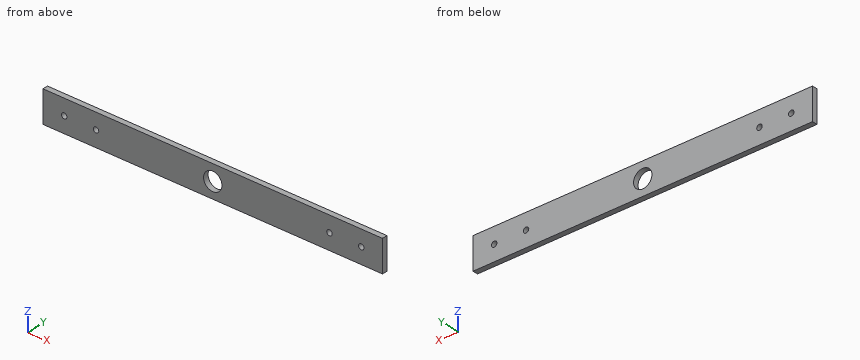
```python
from build123d import *

# Parameters (mm, degrees)
SKETCH1_W                = 406.4
SKETCH1_H                = 38.1
BOSS_EXTRUDE1_DEPTH      = 6.35
SKETCH2_R                = 11
CUT_EXTRUDE1_DEPTH       = 7.62
F_0_257_DIAMETER_HOLE1_D = 6.5278


with BuildPart() as part:
    # Sketch1 → Boss-Extrude1 (new body)
    with BuildSketch(Plane(origin=(0, 0, 0), x_dir=(1, 0, 0), z_dir=(0, 1, 0))):
        Rectangle(SKETCH1_W, SKETCH1_H)
    extrude(amount=BOSS_EXTRUDE1_DEPTH)

    # Sketch2 → Cut-Extrude1 (cut)
    with BuildSketch(Plane(origin=(0, 6.35, 0), x_dir=(1, 0, 0), z_dir=(0, 1, 0))):
        Circle(SKETCH2_R)
    extrude(amount=-CUT_EXTRUDE1_DEPTH, mode=Mode.SUBTRACT)

    # F (0.257) Diameter Hole1 (through all)
    with Locations(Plane(origin=(0, 6.35, 0), x_dir=(1, 0, 0), z_dir=(0, 1, 0))):
        with Locations((177.8, 0), (139.7, 0)):
            f_0_257_diameter_hole1 = Hole(F_0_257_DIAMETER_HOLE1_D / 2)

    # Mirror1: F (0.257) Diameter Hole1 across plane
    add(f_0_257_diameter_hole1.mirror(Plane(origin=(0, 0, 0), x_dir=(0, 0, 1), z_dir=(1, 0, 0))), mode=Mode.SUBTRACT)


solid = part.part
```
CAD build for the part. Positions are in the model's coordinates, mm. Round coordinates to 2 decimals unless told otherwise and drop trailing zeros. Loops run counter-clockwise (first coordinate to the right, second up) from the corner with the lowest first, then second, coordinate; pieces in that order, holes last. Notation, with made-up numbers: (-39, -40) - (-2, -40) arc R5 cw to (-2, -34) - close; hole circle Ø7 at (14.5, -11). An arc over 180 degrees is marked (long way). Return JSON: item names as keys, results as strings. Group by question number.
Q1. Flat gauge pins, fed straight in: pin 1 Ø10.5 at (x, z) = (139.7, 0) entering from +Y; pin 2 Ø6 at (x, z) = (-177.8, 0) entering from +Y. Where does each tip first touch, or does it go through?
Q2. Band-saw the part on A-A on x = 0. Give the cut face in (y, z), plus the area to 3 significant figures.
Q3. Drill centre lines: line 1 along Z through (x, y) = (177.8, 4); line 2 along Z through (x, y) = (0, 3.75); line 3 along X through (y, z) = (1.75, -6.5). Where is each one in solid material? Low to high. Write a range as [from, to].
Q4. Band-saw the part on B-B on y = 3.5. Give the cut face in (x, z).
Solutions:
{
 "1": {"pin 1": "stops at y = 6.35", "pin 2": "passes through"},
 "2": {"outline": "(0, -19.05) - (6.35, -19.05) - (6.35, -11) - (0, -11) - close; (0, 11) - (6.35, 11) - (6.35, 19.05) - (0, 19.05) - close", "area": "102 mm^2"},
 "3": {"line 1": "z = [-19.05, -3.26], [3.26, 19.05]", "line 2": "z = [-19.05, -11], [11, 19.05]", "line 3": "x = [-203.2, -8.87], [8.87, 203.2]"},
 "4": {"outline": "(-203.2, -19.05) - (203.2, -19.05) - (203.2, 19.05) - (-203.2, 19.05) - close; hole circle Ø6.53 at (-177.8, 0); hole circle Ø6.53 at (-139.7, 0); hole circle Ø22 at (0, 0); hole circle Ø6.53 at (139.7, 0); hole circle Ø6.53 at (177.8, 0)"}
}
